Part model, mm, in its own coordinate system. Face numbers are marked on the shaded views. A direction names the side the tool comes from. Coordinates: 2 decimals unless noted, no trailing zeros. Write each loop counter-clockwise with the first axis right and the second up, starting at its lowest first coordinate (ties: lowest second). Pieces come first, ordered by that corner, then holes. Notation, with made-up numbers: (38, -23) -> (67, -23) arc R24 ccw to (67, 8) -> close; hole circle Ø5 at (21.25, 31.5). An arc over 180 degrees is marked (long way). Write item = value, one per line. Start each with the question number.
Q1. Probe line 1 (Z direction, x = 0, y = 2.25); line 2 (Z direction, x = 0, y = 1); line 3 (X direction, y = -1, z = -3). List the from-to ranges inside material, lowest first.
Q2. Band-saw the part on B-B, the plane y = 0. List the corners of the cut face in (x, z).
Q3. Tool access for the marked faces 1 and 2: list every direction of +Z, -Z, +X, -X, +Y, -Y with a clear straight run to the whole face (end or side of a thin tool).
Q4. Band-saw the part on C-C, the plane z = -3.75. List the corners of the cut face in (x, y).
Q5. Pin check, flat tips, straight feed: P1, Ø2, axis at y = 0, z = 4.5, coming from the -X side; P2, Ø3, axis at x = 2, z = 5, coming from the +Y side. Stop position of each tip, or through.
Q6. Band-saw the part on A-A, the plane x = 0. List the corners of the cut face in (y, z), plus the area to 3 significant figures.
Q7. Band-saw the part on D-D, the plane z = 4.25. List the corners of the cut face in (x, y).
Autodesk Inventor part; units mm, degrees
ref_plane "Work Plane1" through (0, 4, 0) normal (0, 1, 0) x (-1, 0, 0)
ref_plane "YZ Plane" through (0, 0, 0) normal (1, 0, 0) x (0, 1, 0)
ref_plane "XY Plane" through (0, 0, 0) normal (0, 0, 1) x (1, 0, 0)
sketch "Sketch1" plane through (0, 0, 0) normal (0, 0, 1) x (1, 0, 0)
  circle A0 centre (0, 0) radius 4
  dimension "d0" = 8
extrude "Extrusion1" add sketch "Sketch1" against normal blind 8
sketch "Sketch2" plane through (0, 0, 0) normal (0, 0, 1) x (1, 0, 0)
  circle A0 centre (0, 0) radius 4
  circle A1 centre (0, 0) radius 1.5
  dimension "d3" = 3
extrude "Extrusion2" add sketch "Sketch2" along normal blind 7 contours A1
thread "Thread1"
fillet "Fillet1" radius 1 1 edges at (-4, 0, -8)
ref_plane "Work Plane1" through (0, 4, 0) normal (0, 1, 0) x (-1, 0, 0)
sketch "Sketch3" plane through (0, 4, 0) normal (0, 1, 0) x (-1, 0, 0)
  line L0 (4, 0) -> (-4, 0)
  line L1 (-4, -7) -> (4, -7)
  arc A0 (0, 0) -> (0, 0) centre (3, -7) ccw
  line L2 (3, -8) -> (-3, -8)
  line L3 (4, 0) -> (4, -7)
  line L4 (-4, 0) -> (-4, -7)
  point P0 (0, -3)
  point P1 (0, -8)
  dimension "d10" = 5
  dimension "d11" = 4
hole "Hole1" at (0, 4, -3) direction (0, -1, 0) diameter 3 end through all
properties part number "33 - Eccentric Swivel Screw" material "Bronze, Soft Tin"
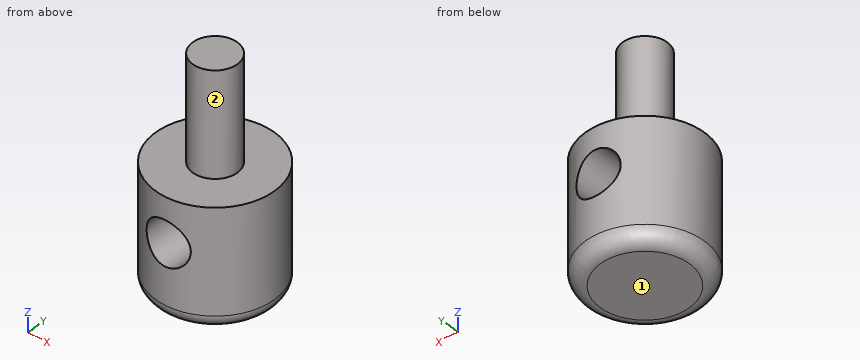
Ans:
q1.line_1 = -8 to -4.5, -1.5 to 0
q1.line_2 = -8 to -4.5, -1.5 to 7
q1.line_3 = -3.87 to -1.5, 1.5 to 3.87
q2.outline = (-4, -7) arc R1 ccw to (-3, -8) -> (3, -8) arc R1 ccw to (4, -7) -> (4, 0) -> (1.5, 0) -> (1.5, 7) -> (-1.5, 7) -> (-1.5, 0) -> (-4, 0) -> close; hole circle Ø3 at (0, -3)
q3.face_1 = -Z, +X, -X, +Y, -Y
q3.face_2 = +Z
q4.outline = (-1.3, -3.78) -> (-1.3, 3.78) arc R4 ccw to start; (1.3, -3.78) arc R4 ccw to (1.3, 3.78) -> close
q5.P1 = -1.5
q5.P2 = 1.41
q6.outline = (-4, -7) arc R1 ccw to (-3, -8) -> (3, -8) arc R1 ccw to (4, -7) -> (4, -4.5) -> (-4, -4.5) -> close; (-4, -1.5) -> (4, -1.5) -> (4, 0) -> (1.5, 0) -> (1.5, 7) -> (-1.5, 7) -> (-1.5, 0) -> (-4, 0) -> close
q6.area = 60.6 mm2
q7.outline = circle Ø3 at (0, 0)
